```python
from build123d import *

# Parameters (mm, degrees)
F0_W     = 1524
F0_H     = 2133.6
F1_DEPTH = 101.6
F2_R     = 38.1
F3_DEPTH = 50.8
F2_W     = 584.2
F2_H     = 304.8
F4_DEPTH = 101.601
F2_W_2   = 685.8
F2_H_2   = 406.4
F5_DEPTH = 25.4


with BuildPart() as f1:
    # F0 (on Right) → F1 (new body)
    with BuildSketch(Plane.YZ):
        with Locations((-868.423025, -6872.774788)):
            Rectangle(F0_W, F0_H)
    extrude(amount=F1_DEPTH)

    # F2 (on face) → F3 (cut)
    with BuildSketch(Plane.YZ.offset(101.6)):
        with Locations((-267.193135, -6896.276238)):
            Circle(F2_R)
    extrude(amount=-F3_DEPTH, mode=Mode.SUBTRACT)

    # F2 (on face) → F4 (cut, through all)
    with BuildSketch(Plane.YZ.offset(101.6)):
        with Locations((-500.123025, -6059.974788)):
            Rectangle(F2_W, F2_H)
        with Locations((-1236.723025, -6059.974788)):
            Rectangle(F2_W, F2_H)
        with Locations((-1236.723025, -6517.174788)):
            Rectangle(F2_W, F2_H)
        with Locations((-500.123025, -6517.174788)):
            Rectangle(F2_W, F2_H)
    extrude(amount=-F4_DEPTH, mode=Mode.SUBTRACT)

    # F2 (on face) → F5 (join)
    with BuildSketch(Plane.YZ.offset(101.6)):
        Polygon((-893.823025, -6313.974788), (-1579.623025, -6313.974788), (-1579.623025, -6720.374788), (-1528.823025, -6720.374788), (-893.823025, -6720.374788), align=None)
        with Locations((-1236.723025, -6517.174788)):
            Rectangle(F2_W, F2_H, mode=Mode.SUBTRACT)
        with Locations((-1236.723025, -6059.974788)):
            Rectangle(F2_W_2, F2_H_2)
        with Locations((-1236.723025, -6059.974788)):
            Rectangle(F2_W, F2_H, mode=Mode.SUBTRACT)
        Polygon((-843.023025, -6313.974788), (-843.023025, -6720.374788), (-208.023025, -6720.374788), (-157.223025, -6720.374788), (-157.223025, -6313.974788), align=None)
        with Locations((-500.123025, -6517.174788)):
            Rectangle(F2_W, F2_H, mode=Mode.SUBTRACT)
        with Locations((-500.123025, -6059.974788)):
            Rectangle(F2_W_2, F2_H_2)
        with Locations((-500.123025, -6059.974788)):
            Rectangle(F2_W, F2_H, mode=Mode.SUBTRACT)
    extrude(amount=F5_DEPTH)


solid = f1.part
```
Here's how the part is built. I have some questions about the finished solid (model axes, mm). A direction names the side the tool comes from. Coordinates: 2 decimals unless noted, no trailing zeros. Order: outer loops, then holes, each group sorted by start corner. A loop starts at its lowest first (then second) coordinate and runs counter-clockwise, first axis right, second up. Notation, with made-up numbers: M 38,65.5 L 92,65.5 A29 ccw 92,94.5 Z; hole C -37.75,-1.5 d6. An arc over 180 degrees is marked long. Answer as a JSON object with one key per item and string values. Group by question number.
(1) Suppose I cut it at B-B, the plane y = -1496. Please give me the cut outline in (x, z), then the cut area to 3 significant figures.
(2) For pin 1 (20.5 mm diameter, centred on x = 116.5, z = -6545.5, fed in from +Y); pin 2 (4 mm diameter, centred on y = -829.5, z = -7420, fed in from +X); pin 3 (20.5 mm diameter, centred on x = 115, z = -5960, fed in from -Y), each with a flat end and sliding along its axis, tell me the tip position at first contact or that it passes through.
(3) If we mould it in two halves opening along Z, with no side actions, what happens to faces 4 (the face through (50, -879, -7939.575)), 5 (the face through (63, -1528.823, -6519)), 6 (the face through (50, -1630.423, -6888))? For each: released by +Z, released by -Z, zero draft, split by the parting line, or undercut.
(4) I need wall thicknesses on probe 1 along Z at (x, y) = (102, -1321); probe 2 along Y at (x, z) = (87, -6585.5); probe 3 along Z at (x, y) = (48.5, -736). Which ranges of each line are inside material? Lowest first, please.
(5) Suppose I cut it at A-A, the plane z = -6401. Please give me the cut outline in (x, y).
(6) Which directions (+Z, -Z, +X, -X, +Y, -Y) give clear straight access to the entire face, cutting with the end or side of a thin tool? Please do faces 1 (the face through (50, -106.423, -6888)), 2 (the face through (64, -504, -5907.575)), 3 (the face through (76.556, -295.274, -6870.526)).
(7) Suppose I cut it at C-C, the plane z = -6802. Please give me the cut outline in (x, y), then the cut area to 3 significant figures.
Values found:
{
 "1": {"outline": "M 0,-7939.57 L 101.6,-7939.57 L 101.6,-6720.37 L 127,-6720.37 L 127,-6669.57 L 0,-6669.57 Z; M 0,-6364.77 L 127,-6364.77 L 127,-6313.97 L 101.6,-6313.97 L 101.6,-6263.17 L 127,-6263.17 L 127,-6212.37 L 0,-6212.37 Z; M 0,-5907.57 L 127,-5907.57 L 127,-5856.77 L 101.6,-5856.77 L 101.6,-5805.97 L 0,-5805.97 Z", "area": "160,000 mm^2"},
 "2": {"pin 1": "stops at y = -157.22", "pin 2": "stops at x = 101.6", "pin 3": "stops at y = -1579.62"},
 "3": {"face 4": "released by -Z", "face 5": "undercut", "face 6": "zero draft"},
 "4": {"probe 1": "z = -6720.37 to -6669.57, -6364.77 to -6313.97, -6263.17 to -6212.37, -5907.57 to -5856.77", "probe 2": "y = -1630.42 to -1528.82, -944.62 to -792.22, -208.02 to -106.42", "probe 3": "z = -7939.57 to -6669.57, -6364.77 to -6212.37, -5907.57 to -5805.97"},
 "5": {"outline": "M 0,-1630.42 L 101.6,-1630.42 L 101.6,-1579.62 L 127,-1579.62 L 127,-1528.82 L 0,-1528.82 Z; M 0,-944.62 L 127,-944.62 L 127,-893.82 L 101.6,-893.82 L 101.6,-843.02 L 127,-843.02 L 127,-792.22 L 0,-792.22 Z; M 0,-208.02 L 127,-208.02 L 127,-157.22 L 101.6,-157.22 L 101.6,-106.42 L 0,-106.42 Z"},
 "6": {"face 1": "+Z, -Z, +X, -X, +Y", "face 2": "+X, -X", "face 3": "+X"},
 "7": {"outline": "M 0,-1630.42 L 101.6,-1630.42 L 101.6,-106.42 L 0,-106.42 Z", "area": "155,000 mm^2"}
}
